Check sheet for the modelled part. Datum: model origin and axes. Units: mm. Give positions to 0.01 mm unless a question says otherwise; leave off trailing zeros. Order: outer loops, then holes, each group sorted by start corner. A loop starts at its lowest first (then second) coordinate and runs counter-clockwise, first axis right, second up. Notation, with made-up numbers: M 34,78.25 L 72,78.25 A20 cw 72,116.25 Z; hole C 49.25,61 d7. An arc over 180 degrees is marked long. Answer in a Markdown table with one row per item. Add a question column.
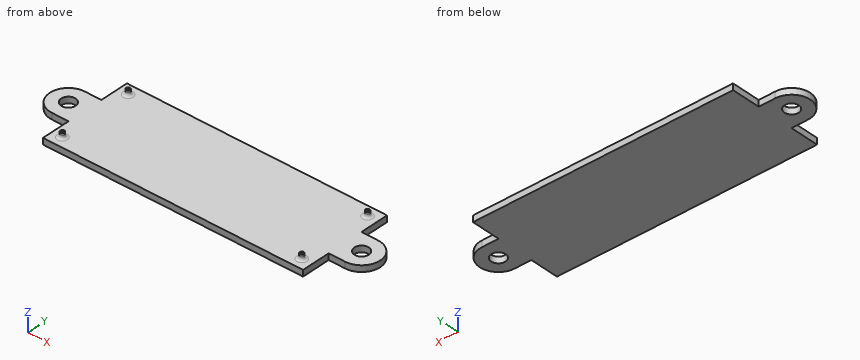
from build123d import *

# Parameters (mm, degrees)
SKETCH_1_W             = 123
SKETCH_1_H             = 43
EXTRUDE_1_DEPTH        = 3
SKETCH_2_W             = 126
SKETCH_2_H             = 46
SKETCH_2_W_2           = 123
SKETCH_2_H_2           = 43
EXTRUDE_2_DEPTH        = 3
SKETCH_5_R             = 1
SKETCH_5_R_2           = 0.697721568
EXTRUDE_5_DEPTH        = 2.5
FILLET_6_R             = 1.5
FILLET_6_OF_MIRROR_1_R = 1.5
SKETCH_8_R             = 3.5
EXTRUDE_8_DEPTH        = 3


# Read off the part's stored shape, not the designer's step: Зеркальное отражение2
with BuildPart() as part:
    # Эскиз1 → Бобышка-Вытянуть1 (new body)
    with BuildSketch(Plane.XY):
        with Locations((61.5, 21.5)):
            Rectangle(SKETCH_1_W, SKETCH_1_H)
    extrude(amount=EXTRUDE_1_DEPTH)

    # Эскиз2 → Бобышка-Вытянуть2 (add)
    with BuildSketch(Plane.XY.offset(3)):
        with Locations((61.5, 21.5)):
            Rectangle(SKETCH_2_W, SKETCH_2_H)
        with Locations((61.5, 21.5)):
            Rectangle(SKETCH_2_W_2, SKETCH_2_H_2, mode=Mode.SUBTRACT)
    extrude(amount=-EXTRUDE_2_DEPTH)

    # Эскиз5 → Бобышка-Вытянуть5 (add)
    with BuildSketch(Plane.XY.offset(3)):
        with Locations(Location((3.5, 39.5, 0), (0, 0, 180))):
            Circle(SKETCH_5_R)
        with Locations((3.5, 39.5)):
            Circle(SKETCH_5_R_2, mode=Mode.SUBTRACT)
    extrude_5 = extrude(amount=EXTRUDE_5_DEPTH)

    # Скругление6
    fillet_6_edges = [part.edges().sort_by_distance(p)[0] for p in [
        (4.5, 39.5, 3),
    ]]
    fillet(fillet_6_edges, radius=FILLET_6_R)

    # Зеркальное отражение1: Бобышка-Вытянуть5 across plane
    add(extrude_5.mirror(Plane.ZY.offset(-61.5)))

    # Скругление6 of Зеркальное отражение1
    fillet_6_of_mirror_1_edges = [part.edges().sort_by_distance(p)[0] for p in [
        (118.5, 39.5, 3),
    ]]
    fillet(fillet_6_of_mirror_1_edges, radius=FILLET_6_OF_MIRROR_1_R)

    # Зеркальное отражение2 outline → Зеркальное отражение2 (revolve)
    with BuildSketch(Plane(origin=(3.5, 3.5, 0), x_dir=(1, 0, 0), z_dir=(0, -1, 0))):
        with BuildLine():
            Line((1, 5.5), (0.697721568, 5.5))
            Line((0.697721568, 5.5), (0.697721568, 3))
            Line((0.697721568, 3), (2.5, 3))
            ThreePointArc((2.5, 3), (1.439339828, 3.439339828), (1, 4.5))
            Line((1, 4.5), (1, 5.5))
        make_face()
    revolve(axis=Axis((3.5, 3.5, 0), (0, 0, 1)))

    # Mirror 2 2 outline → Mirror 2 2 (revolve)
    with BuildSketch(Plane(origin=(119.5, 3.5, 0), x_dir=(1, 0, 0), z_dir=(0, -1, 0))):
        with BuildLine():
            Line((1, 5.5), (0.697721568, 5.5))
            Line((0.697721568, 5.5), (0.697721568, 3))
            Line((0.697721568, 3), (2.5, 3))
            ThreePointArc((2.5, 3), (1.439339828, 3.439339828), (1, 4.5))
            Line((1, 4.5), (1, 5.5))
        make_face()
    revolve(axis=Axis((119.5, 3.5, 0), (0, 0, 1)))

    # Эскиз8 → Бобышка-Вытянуть8 (add)
    with BuildSketch(Plane(origin=(0, 0, 0), x_dir=(-1, 0, 0), z_dir=(0, 0, -1))):
        with BuildLine():
            Line((-124.5, 12.5), (-132.54002612, 12.5))
            ThreePointArc((-132.54002612, 12.5), (-141.54002612, 21.5), (-132.54002612, 30.5))
            Line((-132.54002612, 30.5), (-124.5, 30.5))
            Line((-124.5, 30.5), (-124.5, 12.5))
        make_face()
        with Locations((-132.54002612, 21.5)):
            Circle(SKETCH_8_R, mode=Mode.SUBTRACT)
    extrude_8 = extrude(amount=-EXTRUDE_8_DEPTH)

    # Зеркальное отражение8: Бобышка-Вытянуть8 across plane
    add(extrude_8.mirror(Plane.ZY.offset(-61.5)))


solid = part.part
Q1. Cross-section at B-B (z = 0.9). Record the boundary of the cut face in (x, y), and give its area (3 significant figures).
Q2. Go/stop test with flat-tipped pins: pin 1 (2.5 mm diameter, centred on x = 129.5, z = 1, fed in from -Y); pin 2 (1.5 mm diameter, centred on y = 3, z = 2, fed in from +X); pin 3 (3 mm diameter, centred on y = 26, z = 3.5, fed in from +X). Record where each tip stops, or that it passes through.
Q3. Cross-section at A-A (y = 21.5). Record the boundary of the cut face in (x, z).
Q4. Thickness scan on probe 1 along X at (y, z) = (39.5, 4.2); probe 2 along Y at (x, z) = (119.5, 4.3); probe 3 along Z at (x, y) = (94.5, 24). Record the ranges inside material, lowest first.
Q5. Cross-section at C-C (x = -3). Record the boundary of the cut face in (y, z), and give its area (3 significant figures).
Q6. Cross-section at D-D (x = 17). Record the boundary of the cut face in (y, z).
Values follow:
| question | item | result |
|---|---|---|
| 1 | outline | M -9.54,12.5 L -1.5,12.5 L -1.5,-1.5 L 124.5,-1.5 L 124.5,12.5 L 132.54,12.5 A9 ccw 132.54,30.5 L 124.5,30.5 L 124.5,44.5 L -1.5,44.5 L -1.5,30.5 L -9.54,30.5 A9 ccw Z; hole C -9.54,21.5 d7; hole C 132.54,21.5 d7 |
| 1 | area | 6,260 mm² |
| 2 | pin 1 | y = 12.5 |
| 2 | pin 2 | x = 124.5 |
| 2 | pin 3 | x = 140.99 |
| 3 | outline | M -18.54,0 L -13.04,0 L -13.04,3 L -18.54,3 Z; M -6.04,0 L 129.04,0 L 129.04,3 L -6.04,3 Z; M 136.04,0 L 141.54,0 L 141.54,3 L 136.04,3 Z |
| 4 | probe 1 | 2.47 to 2.8, 4.2 to 4.53, 118.47 to 118.8, 120.2 to 120.53 |
| 4 | probe 2 | 2.49 to 2.8, 4.2 to 4.51, 38.49 to 38.8, 40.2 to 40.51 |
| 4 | probe 3 | 0 to 3 |
| 5 | outline | M 12.5,0 L 30.5,0 L 30.5,3 L 12.5,3 Z |
| 5 | area | 54.0 mm² |
| 6 | outline | M -1.5,0 L 44.5,0 L 44.5,3 L -1.5,3 Z |
